Can you work these out from the model? Positions are in its coordinate system, mm. Coordinates: 2 decimals unless noted, no trailing zeros. Order: outer loops, then holes, each group sorted by start corner. A loop starts at its lowest first (then second) coordinate and runs counter-clockwise, first axis right, second up. Notation, with made-up numbers: (1, -28) -> (28, -28) arc R25 ccw to (28, -4) -> close; hole circle Ø2 at (25, 2.25). An arc over 180 degrees is marked (long way). Use a Markdown table: item, result. Add a question column.
1. For pin 1 Ø12 at (y, z) = (-47.5, 292) entering from -X; pin 2 Ø12 at (x, z) = (-38.5, 328.5) entering from -Y; pin 3 Ø11 at (y, z) = (-28, -424) entering from +X, each with a flat end and sliding along its axis, tell me the tip position at first contact or that it passes through.
2. If I drill on line 1 along X through (y, z) = (1.5, -247); line 2 along Z through (x, y) = (35, 0); line 3 along Y through (x, z) = (0, -235), over which ranges is the centre line in solid material (lowest first)? Write a range as from..to.
3. Suppose I cut it at B-B, the plane z = 203.5. List the corners of the cut face in (x, y) for me.
4. Suppose I cut it at A-A, the plane y = 0. List the corners of the cut face in (x, z) for me.
```python
from build123d import *

# Parameters (mm, degrees)
F0_R     = 60
F0_R_2   = 25
F1_DEPTH = 500
F3_D     = 70
F3_DEPTH = 60.001
F5_D     = 70
F5_DEPTH = 60.0010001


with BuildPart() as f1:
    # F0 (on Top) → F1 (new body, symmetric)
    with BuildSketch(Plane.XY):
        Circle(F0_R)
        Circle(F0_R_2, mode=Mode.SUBTRACT)
    extrude(amount=F1_DEPTH, both=True)

    # F3 (through all, one way)
    with BuildSketch(Plane.YZ):
        with Locations((0, 433.1713616848)):
            Circle(F3_D / 2)
    extrude(amount=-F3_DEPTH, mode=Mode.SUBTRACT)

    # F5 (through all, one way)
    with BuildSketch(Plane(origin=(0, 0, 0), x_dir=(0, 1, 0), z_dir=(-1, 0, 0))):
        with Locations((0, 423.8957464695)):
            Circle(F5_D / 2)
    extrude(amount=-F5_DEPTH, mode=Mode.SUBTRACT)


solid = f1.part
```
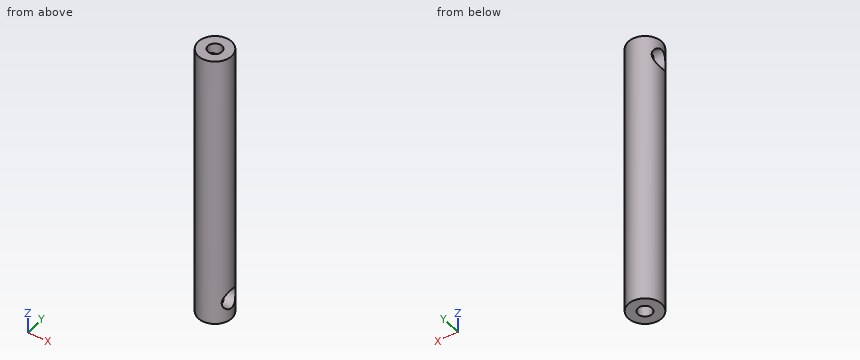
Worked out:
| question | item | result |
|---|---|---|
| 1 | pin 1 | stops at x = -43.33 |
| 1 | pin 2 | stops at y = -50.44 |
| 1 | pin 3 | stops at x = 0 |
| 2 | line 1 | x = -59.98..-24.95, 24.95..59.98 |
| 2 | line 2 | z = -500..-458.9, -388.9..500 |
| 2 | line 3 | y = -60..-25, 25..60 |
| 3 | outline | circle Ø120 at (0, 0); hole circle Ø50 at (0, 0) |
| 4 | outline | (-60, -500) -> (-25, -500) -> (-25, 398.17) -> (-60, 398.17) -> close; (-60, 468.17) -> (-25, 468.17) -> (-25, 500) -> (-60, 500) -> close; (25, -500) -> (60, -500) -> (60, -458.9) -> (25, -458.9) -> close; (25, -388.9) -> (60, -388.9) -> (60, 500) -> (25, 500) -> close |
